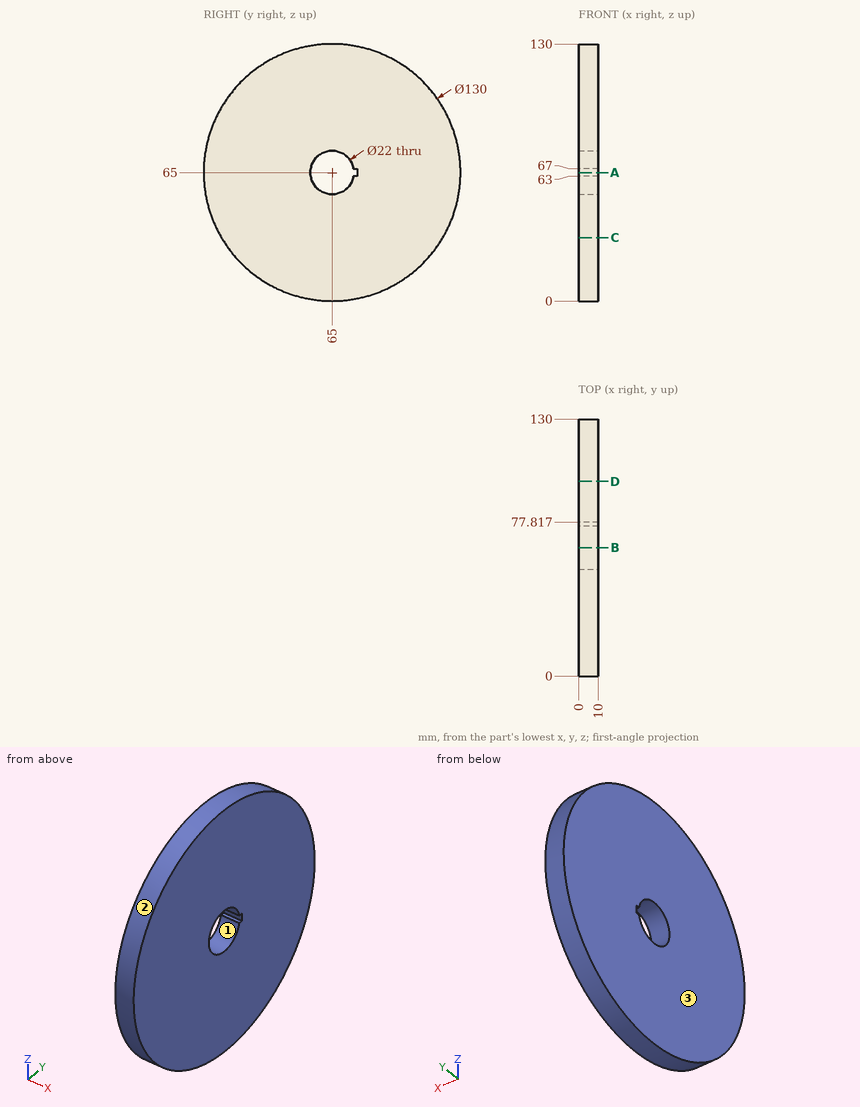
Verification items for this drawing (mm, ordinates from the low corner). Give positions to 0.01 mm unless a question says otherwise; leave off trailing zeros. Loops run counter-clockwise (first coordinate to the right, second up) from the corner with the lowest first, then second, coordinate; pieces in that order, holes last. Notation, with made-up numbers: M -9,-1.75 L 43,-1.75 A7 ccw 43,11.25 Z; hole C 48,46.25 d8. An arc over 180 degrees is marked long. Answer as CSV lines item,"result".
Item 1: Depth check by flat-ended pin: P1, Ø0.6, axis at x = 5.5, y = 76.5, coming from the +Z side; P2, Ø1, axis at x = 6, y = 24, coming from the -Z side; P3, Ø1.5, axis at x = 8.5, z = 27, coming from the -Y side. Enter the tip coordinate at first touch or a pass-through.
Values:
P1,"stops at z = 129.03"
P2,"stops at z = 14.16"
P3,"stops at y = 11.73"
Item 2: Cross-section at C-C on z = 32. Record the cut outline in (x, y).
Values:
outline,"M 0,9 L 10,9 L 10,121 L 0,121 Z"
Item 3: Cross-section at D-D on y = 98.5. Record the cut outline in (x, z).
Values:
outline,"M 0,9.3 L 10,9.3 L 10,120.7 L 0,120.7 Z"
Item 4: Release check for a two-part mould opening along Y. For the marked faces 1, 2 and 3 record: pulls with the +Y half, pulls with the -Y half, needs draft (parallel to the pull), parting line crosses it, or undercut.
Values:
face 1,"undercut"
face 2,"parting line crosses it"
face 3,"needs draft"
Item 5: Cross-section at A-A on z = 65. Record the cut outline in (x, y).
Values:
outline,"M 0,0 L 10,0 L 10,54 L 0,54 Z; M 0,77.82 L 10,77.82 L 10,130 L 0,130 Z"
Item 6: Cross-section at B-B on y = 65. Record the cut outline in (x, z), and give its area (3 significant figures).
Values:
outline,"M 0,0 L 10,0 L 10,54 L 0,54 Z; M 0,76 L 10,76 L 10,130 L 0,130 Z"
area,"1,080 mm²"
Item 7: Material ranges on line 1 (Y direction, x = 5.25, z = 65); line 2 (Y direction, x = 9.5, z = 58.5) (1 decimal); line 3 (Y direction, x = 8.75, z = 53), recorded low to high.
Values:
line 1,"y = 0 to 54, 77.82 to 130"
line 2,"y = 0.3 to 56.1, 73.9 to 129.7"
line 3,"y = 1.12 to 128.88"
